```python
from build123d import *

# Parameters (mm, degrees)
SKETCH053_W             = 40
SKETCH053_H             = 15
PAD031_DEPTH            = 10
POCKET022_DEPTH         = 10
SKETCH051_W             = 20
SKETCH051_H             = 20
PAD030_DEPTH            = 30
SKETCH058_R             = 3
POCKET023_DEPTH         = 250
SKETCH052_W             = 7
SKETCH052_H             = 10
POCKET024_DEPTH         = 27
SKETCH055_W             = 10
SKETCH055_H             = 10
POCKET021_DEPTH         = 20
FILLET004_R             = 4
SKETCH057_W             = 5
SKETCH057_H             = 5
POCKET025_DEPTH         = 25
SKETCH008_W             = 12
SKETCH008_H             = 12
POCKET005_DEPTH         = 17.5
BODY016_PLACEMENT_ANGLE = 285


with BuildPart() as part:
    # Sketch053 → Pad031 (new body, symmetric)
    with BuildSketch(Plane.XZ):
        with Locations((-10, 7.5)):
            Rectangle(SKETCH053_W, SKETCH053_H)
    extrude(amount=PAD031_DEPTH, both=True)

    # Sketch056 → Pocket022 (cut)
    with BuildSketch(Plane.XY):
        Polygon((-25.2, 5.1), (-30.2, 5.1), (-30.2, -5.1), (-25.2, -5.1), (-25.2, -10), (-15, -10), (-15, 10), (-25.2, 10), align=None)
    extrude(amount=POCKET022_DEPTH, mode=Mode.SUBTRACT)

    # Sketch051 → Pad030 (join)
    with BuildSketch(Plane.XY):
        Rectangle(SKETCH051_W, SKETCH051_H)
    extrude(amount=PAD030_DEPTH)

    # Sketch058 → Pocket023 (cut, symmetric)
    with BuildSketch(Plane.XY):
        Circle(SKETCH058_R)
    extrude(amount=POCKET023_DEPTH, both=True, mode=Mode.SUBTRACT)

    # Sketch052 → Pocket024 (cut)
    with BuildSketch(Plane.XY):
        Rectangle(SKETCH052_W, SKETCH052_H)
    extrude(amount=POCKET024_DEPTH, mode=Mode.SUBTRACT)

    # Sketch055 → Pocket021 (cut)
    with BuildSketch(Plane.YZ):
        with Locations((0, 5)):
            Rectangle(SKETCH055_W, SKETCH055_H)
    extrude(amount=-POCKET021_DEPTH, mode=Mode.SUBTRACT)

    # Fillet004
    fillet004_edges = [part.edges().sort_by_distance(p)[0] for p in [
        (0, -10, 30),
        (10, 0, 30),
        (-10, 0, 30),
        (0, 10, 30),
    ]]
    fillet(fillet004_edges, radius=FILLET004_R)

    # Sketch057 → Pocket025 (cut, symmetric)
    with BuildSketch(Plane.XZ):
        with Locations((0, 7.5)):
            Rectangle(SKETCH057_W, SKETCH057_H)
    extrude(amount=POCKET025_DEPTH, both=True, mode=Mode.SUBTRACT)

    # Sketch008 → Pocket005 (cut, symmetric)
    with BuildSketch(Plane.XY):
        Rectangle(SKETCH008_W, SKETCH008_H)
    extrude(amount=POCKET005_DEPTH, both=True, mode=Mode.SUBTRACT)


with BuildPart() as part_1:
    # Body016 placement: moved
    add(part.part.moved(Location((191, -1.478585, -56.301099))).rotate(Axis((191, -1.478585, -56.301099), (1, 0, 0)), BODY016_PLACEMENT_ANGLE))


solid = part_1.part
```
Source: CAD feature listing. Evaluate the final solid. Frame: model axes, mm. A direction names the side the tool comes from. Coordinates: 2 decimals unless noted, no trailing zeros. Write each loop counter-clockwise with the first axis right and the second up, starting at its lowest first coordinate (ties: lowest second). Pieces come first, ordered by that corner, then holes. Notation, with made-up numbers: (72, 28) - (104, 28) arc R17 ccw to (104, 42) - close; hole circle Ø10 at (30.25, 85.25). An arc over 180 degrees is marked (long way). Answer as a JSON object with one key per item and string values.
Q1. Section query D-D, the plane y = 8.5. Output: boundary loops of the cut face in (x, z).
Ans:
{"outline": "(161, -63.98) - (165.8, -63.98) - (165.8, -58.91) - (161, -58.91) - close; (161, -54.9) - (185, -54.9) - (185, -47.42) - (197, -47.42) - (197, -59.84) - (193.5, -59.84) - (193.5, -63.98) - (201, -63.98) - (201, -43.27) - (161, -43.27) - close; (176, -63.98) - (188.5, -63.98) - (188.5, -59.84) - (185, -59.84) - (185, -58.8) - (176, -58.8) - close"}
Q2. Material intervals for line 1 (X direction, y = 2, z = -65); line 2 (X direction, y = 16.5, z = -48.25); line 3 (Z direction, x = 185.5, y = 6), sorted ascending. Write a range as [from, to].
Ans:
{"line 1": "x = [161, 165.8], [176, 201]", "line 2": "x = [181, 187.5], [194.5, 201]", "line 3": "z = [-64.65, -60.51], [-48.09, -43.94]"}
Q3. Draft query along Y for faces 6 (the cylindrical face through (191.14, 24.04, -40.29)), 7 (the flat face through (193.5, 4, -47)), 8 (the flat face through (188.32, -3.24, -49.73)). Return one class per face: released by +Y, released by -Y, zero draft, split by the parting line, or undercut.
Ans:
{"face 6": "split by the parting line", "face 7": "undercut", "face 8": "released by -Y"}
Q4. Section query C-C, the plane z = -60. Output: boundary loops of the cut face in (x, y).
Ans:
{"outline": "(161, 4.42) - (165.8, 4.42) - (165.8, 9.87) - (176, 9.87) - (176, 4.04) - (185, 4.04) - (185, 7.9) - (188.5, 7.9) - (188.5, 9.87) - (193.5, 9.87) - (193.5, 7.9) - (197, 7.9) - (197, -0.49) - (201, -0.49) - (201, 23.35) - (181, 23.35) - (181, 15.04) - (161, 15.04) - close"}
Q5. Set-up query: faces 1 (the flat face through (187.84, 24.62, -49.38)), 2 (the flat face through (180.563, 1.989, -50.195)), 3 (the flat face through (163.434, 4.603, -59.951)), 4 (the flat face through (190.965, 1.273, -47.253)), 5 (the flat face through (170.86, 12.974, -52.284)). Return all of +Z, -Z, +X, -X, +Y, -Y with unobstructed straight access to the full face (end or side cutting, diameter ignored); none if empty.
Ans:
{"face 1": "none", "face 2": "-X", "face 3": "-X, -Y", "face 4": "+Z", "face 5": "+Z, -X, +Y"}
Q6. Section query B-B, the plane x = 179.5. Output: boundary loops of the cut face in (y, z).
Ans:
{"outline": "(-4.07, -46.64) - (-2.77, -51.47) - (6.89, -48.88) - (9.47, -58.54) - (-0.18, -61.13) - (1.11, -65.96) - (15.6, -62.08) - (10.42, -42.76) - close"}
Q7. Section query A-A, the plane y = 3.5. Output: boundary loops of the cut face in (x, z), plus the area to 3 significant figures.
Ans:
{"outline": "(161, -65.32) - (165.8, -65.32) - (165.8, -60.25) - (161, -60.25) - close; (161, -49.69) - (165.8, -49.69) - (165.8, -44.61) - (161, -44.61) - close; (176, -65.32) - (201, -65.32) - (201, -44.61) - (193.5, -44.61) - (193.5, -48.76) - (197, -48.76) - (197, -61.18) - (185, -61.18) - (185, -60.14) - (176, -60.14) - close; (176, -49.79) - (185, -49.79) - (185, -48.76) - (188.5, -48.76) - (188.5, -44.61) - (176, -44.61) - close", "area": "303 mm2"}
Q8. First-contact query: pin 1 Ø4 at (x, y) = (184.5, 6.5) entering from +Z; pin 2 Ø1.5 at (x, y) = (170.5, 5) entering from +Z; pin 3 Ø6 at (x, z) = (166.5, -56) entering from -Y. Flat tips, straight axial feed; report the tip coordinate or a pass-through.
Ans:
{"pin 1": "stops at z = -43.27", "pin 2": "stops at z = -44.01", "pin 3": "stops at y = 7.99"}
